The listing builds one solid part. Answer for the finished solid, in the listing's coordinates (mm). A direction names the side the tool comes from. Round coordinates to 2 decimals unless told otherwise and drop trailing zeros. Order: outer loops, then holes, each group sorted by start corner. A loop starts at its lowest first (then second) coordinate and runs counter-clockwise, first axis right, second up. Notation, with made-up numbers: (65, 9.25) -> (109, 9.25) arc R9 ccw to (109, 22.25) -> close; hole circle Ø10 at (6.25, -27.75). An arc over 180 degrees is marked (long way). Answer in a Markdown table with one row per item. Add a question column.
```python
from build123d import *

# Parameters (mm, degrees)
EXTRUDE_1_DEPTH             = 54
EXTRUDE_2_DEPTH             = 25
HOLE_WIZARD_M31_D           = 3.4
HOLE_WIZARD_M31_CBORE_D     = 6.5
HOLE_WIZARD_M31_CBORE_DEPTH = 3
SKETCH_6_W                  = 16
SKETCH_6_H                  = 16
EXTRUDE_3_DEPTH             = 18
HOLE_WIZARD_M32_D           = 3.4
HOLE_WIZARD_M32_CBORE_D     = 6.5
HOLE_WIZARD_M32_CBORE_DEPTH = 3


with BuildPart() as part:
    # Эскиз1 → Бобышка-Вытянуть1 (new body)
    with BuildSketch(Plane.XY):
        Polygon((0, 0), (0, 11), (12, 11), (12, 7), (8, 7), (8, 3), (38, 3), (38, 7), (34, 7), (34, 11), (46, 11), (46, 0), align=None)
    extrude(amount=EXTRUDE_1_DEPTH)

    # Эскиз2 → Бобышка-Вытянуть2 (add)
    with BuildSketch(Plane.XY.offset(54)):
        Polygon((0, 11), (12, 11), (34, 11), (46, 11), (46, 0), (0, 0), align=None)
    extrude(amount=EXTRUDE_2_DEPTH)

    # Цековка для винта с внутренним шестигранником M31 (through all)
    with Locations(Plane(origin=(0, 11, 0), x_dir=(1, 0, 0), z_dir=(0, 1, 0))):
        with Locations((42, -4), (42, -75), (4, -4), (4, -75)):
            CounterBoreHole(HOLE_WIZARD_M31_D / 2, HOLE_WIZARD_M31_CBORE_D / 2, HOLE_WIZARD_M31_CBORE_DEPTH)

    # Эскиз6 → Бобышка-Вытянуть3 (add)
    with BuildSketch(Plane(origin=(0, 11, 0), x_dir=(1, 0, 0), z_dir=(0, 1, 0))):
        with Locations((23, -71)):
            Rectangle(SKETCH_6_W, SKETCH_6_H)
    extrude(amount=EXTRUDE_3_DEPTH)

    # Цековка для винта с внутренним шестигранником M32 (through all)
    with Locations(Plane.XY.offset(79)):
        with Locations((23, 21)):
            CounterBoreHole(HOLE_WIZARD_M32_D / 2, HOLE_WIZARD_M32_CBORE_D / 2, HOLE_WIZARD_M32_CBORE_DEPTH)


solid = part.part
```
1. The part is cut by section B-B (z = 75). Give the vertices of the cut face in (x, y), then the cut area to 3 significant figures.
2. The part is cut by section D-D (x = 23). Give the vertices of the cut face in (y, z).
3. Straight lines are drawn through the part: line 1 along Z through (x, y) = (42, 5); line 2 along X through (y, z) = (4.75, 4); line 3 along X through (y, z) = (4, 15.5). For each, find the intervals that lie inside material, in ascending order.
4. The mould has two halves that part along X. Classify faces 6 (the flat face through (31, 20, 71)), 7 (the flat face through (12, 9, 27)), 8 (the flat face through (21, 20, 63)): released by +X, released by -X, zero draft, split by the parting line, or undercut.
5. The part is cut by section C-C (z = 4). Give the vertices of the cut face in (x, y).
6. The part is cut by section A-A (x = 4). Give the vertices of the cut face in (y, z), then the cut area to 3 significant figures.
7. For faces 1 (the flat face through (5.4, 8, 5.4)), 2 (the flat face through (10, 7, 27)), 3 (the flat face through (34, 9, 27)), 4 (the flat face through (23, 0, 39)), 5 (the cylindrical face through (20.421, 19.022, 77.521)), determine the directions among +Z, -Z, +X, -X, +Y, -Y from which every point of the face is accessible in a straight line to the end or side of a thin tool.
8. Each of these flat-tipped pins is pushed along its axis until it touches: pin 1 (4.5 mm diameter, centred on x = 42, z = 75, fed in from +Y); pin 2 (4 mm diameter, centred on y = 21, z = 65, fed in from -X); pin 3 (1.5 mm diameter, centred on x = 23, y = 7, fed in from -Z). Where does it stop, or does it pass through?
Report:
| question | item | result |
|---|---|---|
| 1 | outline | (0, 0) -> (2.3, 0) -> (2.3, 8) -> (0.75, 8) -> (0.75, 11) -> (0, 11) -> close; (5.7, 0) -> (40.3, 0) -> (40.3, 8) -> (38.75, 8) -> (38.75, 11) -> (31, 11) -> (31, 29) -> (15, 29) -> (15, 11) -> (7.25, 11) -> (7.25, 8) -> (5.7, 8) -> close; (43.7, 0) -> (46, 0) -> (46, 11) -> (45.25, 11) -> (45.25, 8) -> (43.7, 8) -> close; hole circle Ø3.4 at (23, 21) |
| 1 | area | 692 mm^2 |
| 2 | outline | (0, 0) -> (3, 0) -> (3, 54) -> (11, 54) -> (11, 63) -> (19.3, 63) -> (19.3, 76) -> (17.75, 76) -> (17.75, 79) -> (0, 79) -> close; (22.7, 63) -> (29, 63) -> (29, 79) -> (24.25, 79) -> (24.25, 76) -> (22.7, 76) -> close |
| 3 | line 1 | z = 0 to 2.3, 5.7 to 73.3, 76.7 to 79 |
| 3 | line 2 | x = 0 to 2.3, 5.7 to 8, 38 to 40.3, 43.7 to 46 |
| 3 | line 3 | x = 0 to 8, 38 to 46 |
| 4 | face 6 | released by +X |
| 4 | face 7 | undercut |
| 4 | face 8 | zero draft |
| 5 | outline | (0, 0) -> (2.3, 0) -> (2.3, 8) -> (0.75, 8) -> (0.75, 11) -> (0, 11) -> close; (5.7, 0) -> (40.3, 0) -> (40.3, 8) -> (38.75, 8) -> (38.75, 11) -> (34, 11) -> (34, 7) -> (38, 7) -> (38, 3) -> (8, 3) -> (8, 7) -> (12, 7) -> (12, 11) -> (7.25, 11) -> (7.25, 8) -> (5.7, 8) -> close; (43.7, 0) -> (46, 0) -> (46, 11) -> (45.25, 11) -> (45.25, 8) -> (43.7, 8) -> close |
| 6 | outline | (0, 0) -> (11, 0) -> (11, 0.75) -> (8, 0.75) -> (8, 2.3) -> (0, 2.3) -> close; (0, 5.7) -> (8, 5.7) -> (8, 7.25) -> (11, 7.25) -> (11, 71.75) -> (8, 71.75) -> (8, 73.3) -> (0, 73.3) -> close; (0, 76.7) -> (8, 76.7) -> (8, 78.25) -> (11, 78.25) -> (11, 79) -> (0, 79) -> close |
| 6 | area | 776 mm^2 |
| 7 | face 1 | +Y |
| 7 | face 2 | -Z |
| 7 | face 3 | -Z, +Y |
| 7 | face 4 | +Z, -Z, +X, -X, -Y |
| 7 | face 5 | +Z |
| 8 | pin 1 | stops at y = 8 |
| 8 | pin 2 | stops at x = 15 |
| 8 | pin 3 | stops at z = 54 |
